from build123d import *

# Parameters (mm, degrees)
F0_R     = 1.651
F0_W     = 2.54
F0_H     = 13.97
F1_DEPTH = 2.032
F2_R     = 1.651
F3_DEPTH = 3.302
F4_R     = 2.54
F5_DEPTH = 1.524
F6_R     = 2.794
F7_DEPTH = 4.572
F8_R     = 1.14299


# Not quite as in the source:
# - a fillet or chamfer is up to 0.001 mm smaller than in the source, because OpenCascade refuses the exact size


with BuildPart() as f1:
    # F0 (on Top) → F1 (new body)
    with BuildSketch(Plane.XY):
        with BuildLine():
            Line((42.545, 3.81), (-76.835, 3.81))
            ThreePointArc((-76.835, 3.81), (-80.645, 0), (-76.835, -3.81))
            Line((-76.835, -3.81), (42.545, -3.81))
            Line((42.545, -3.81), (45.2222972973, -11.6187837838))
            ThreePointArc((45.2222972973, -11.6187837838), (47.625, -13.335), (50.0277027027, -11.6187837838))
            Line((50.0277027027, -11.6187837838), (52.705, -3.81))
            Line((52.705, -3.81), (59.055, -3.81))
            Line((59.055, -3.81), (59.055, -10.16))
            ThreePointArc((59.055, -10.16), (62.865, -13.97), (66.675, -10.16))
            Line((66.675, -10.16), (66.675, -3.81))
            Line((66.675, -3.81), (76.835, -3.81))
            ThreePointArc((76.835, -3.81), (80.645, 0), (76.835, 3.81))
            Line((76.835, 3.81), (66.675, 3.81))
            Line((66.675, 3.81), (66.675, 10.16))
            ThreePointArc((66.675, 10.16), (62.865, 13.97), (59.055, 10.16))
            Line((59.055, 10.16), (59.055, 3.81))
            Line((59.055, 3.81), (52.705, 3.81))
            Line((52.705, 3.81), (50.0277027027, 11.6187837838))
            ThreePointArc((50.0277027027, 11.6187837838), (47.625, 13.335), (45.2222972973, 11.6187837838))
            Line((45.2222972973, 11.6187837838), (42.545, 3.81))
        make_face()
        with Locations((-76.835, 0)):
            Circle(F0_R, mode=Mode.SUBTRACT)
        with Locations((-36.195, 0)):
            Circle(F0_R, mode=Mode.SUBTRACT)
        with Locations((62.865, -10.16)):
            Circle(F0_R, mode=Mode.SUBTRACT)
        with Locations((47.625, 0)):
            Circle(F0_R, mode=Mode.SUBTRACT)
        with Locations((62.865, 0)):
            Rectangle(F0_W, F0_H, mode=Mode.SUBTRACT)
        with Locations((76.835, 0)):
            Circle(F0_R, mode=Mode.SUBTRACT)
        with Locations((62.865, 10.16)):
            Circle(F0_R, mode=Mode.SUBTRACT)
    extrude(amount=F1_DEPTH)

    # F2 (on face) → F3 (join)
    with BuildSketch(Plane.XY.offset(2.032)):
        with BuildLine():
            ThreePointArc((50.0277027027, 11.6187837838), (47.625, 13.335), (45.2222972973, 11.6187837838))
            Line((45.2222972973, 11.6187837838), (42.545, 3.81))
            Line((42.545, 3.81), (42.545, -3.81))
            Line((42.545, -3.81), (45.2222972973, -11.6187837838))
            ThreePointArc((45.2222972973, -11.6187837838), (47.625, -13.335), (50.0277027027, -11.6187837838))
            Line((50.0277027027, -11.6187837838), (52.705, -3.81))
            Line((52.705, -3.81), (52.705, 3.81))
            Line((52.705, 3.81), (50.0277027027, 11.6187837838))
        make_face()
        with Locations((47.625, 0)):
            Circle(F2_R, mode=Mode.SUBTRACT)
    extrude(amount=F3_DEPTH)

    # F4 (on face) → F5 (join)
    with BuildSketch(Plane.XY.offset(5.334)):
        with Locations((47.625, 10.795)):
            Circle(F4_R)
        with Locations((47.625, -10.795)):
            Circle(F4_R)
    extrude(amount=F5_DEPTH)

    # F6 (on face) → F7 (cut)
    with BuildSketch(Plane(origin=(0, 0, 0), x_dir=(1, 0, 0), z_dir=(0, 0, -1))):
        with Locations((47.625, 0)):
            Circle(F6_R)
    extrude(amount=-F7_DEPTH, mode=Mode.SUBTRACT)

    # F8 (radius 1.143 in the source; OpenCascade refuses exactly that, so slightly less here)
    f8_edges = [f1.edges().sort_by_distance(p)[0] for p in [
        (44.831, 0, 4.572),
    ]]
    fillet(f8_edges, radius=F8_R)


solid = f1.part
The model under review builds one solid part; all positions refer to its coordinate system, in mm. A direction names the side the tool comes from. Coordinates: 2 decimals unless noted, no trailing zeros. Write each loop counter-clockwise with the first axis right and the second up, starting at its lowest first coordinate (ties: lowest second). Pieces come first, ordered by that corner, then holes. Notation, with made-up numbers: (-29.75, 36) - (5.25, 36) arc R32 cw to (5.25, 72) - close; hole circle Ø2 at (21.25, 51). An arc over 180 degrees is marked (long way). Answer as a JSON object with one key per item and string values. Group by question number.
1. Add section A-A (y = 0). Give the number of separate pieces and of enclosed holes in the cut face, plus the area to 3 significant figures.
2. Add section B-B (x = -4.5). Give the boundary of the cut face in (y, z).
3. Machinability: for faces 1 (the face through (51.385, 7.66, 2.63)), 2 (the face through (80.644, -0.084, 1.002)), 3 (the face through (51.348, -7.769, 2.63)), 4 (the face through (50.3, -0.8, 1.7)), 5 (the face through (-20, 0, 2.032)), which of the approach directions +Z, -Z, +X, -X, +Y, -Y give a long, thin tool a straight path to every point of the face, cutting with its end or side? Answer none if there is none.
4. To check wall thickness, follow probe 1 along Z at (x, y) = (50, -2); probe 2 along Z at (x, y) = (42.5, 3.25); probe 3 along Y at (x, z) = (71, 2). State the ranges of each line that lie inside material, in increasing order.
5. Mouldability with a two-part tool opening along X and no side actions: class faces 6 (the face through (50, 0, 5.334)), 7 (the face through (43.865, -7.66, 2.63)), 8 (the face through (52.705, 0, 4)), 9 (the face through (75.186, 0.073, 1.002)) as pulls with the +X half, pulls with the -X half, needs draft (parallel to the pull), parting line crosses it, or undercut.
6. Clearance check with flat-ended pins moving along their axes: pin 1 Ø4 at (x, z) = (51, 3.5) entering from -Y; pin 2 Ø2 at (y, z) = (-8, 0.5) entering from -X; pin 3 Ø1 at (x, y) = (-10, 0) entering from +Z; pin 4 Ø0.6 at (x, z) = (63, 1.5) entering from +Y. State where each tip first meets the part, or that it passes through.
Findings:
{
 "1": {"separate pieces": "6", "enclosed holes": "0", "area": "308 mm²"},
 "2": {"outline": "(-3.81, 0) - (3.81, 0) - (3.81, 2.03) - (-3.81, 2.03) - close"},
 "3": {"face 1": "+Z, -Z, +Y", "face 2": "+Z, -Z, +X", "face 3": "+Z, -Z, -Y", "face 4": "-Z", "face 5": "+Z, -X, +Y, -Y"},
 "4": {"probe 1": "0 to 5.33", "probe 2": "0 to 2.03", "probe 3": "-3.81 to 3.81"},
 "5": {"face 6": "needs draft", "face 7": "pulls with the -X half", "face 8": "pulls with the +X half", "face 9": "undercut"},
 "6": {"pin 1": "y = -12.93", "pin 2": "x = 43.64", "pin 3": "z = 2.03", "pin 4": "y = 13.97"}
}
